from build123d import *

# Parameters (mm, degrees)
CROQUIS4_R                  = 2.5
SALIENTE_EXTRUIR1_DEPTH     = 4
CROQUIS5_R                  = 21
SALIENTE_EXTRUIR2_DEPTH     = 8.5
SALIENTE_EXTRUIR4_START     = -3
SALIENTE_EXTRUIR4_DEPTH     = 3
REDONDEO1_R                 = 10
SALIENTE_EXTRUIR5_OUTLINE_R = 2
SALIENTE_EXTRUIR5_DEPTH     = 15
CROQUIS9_R                  = 1.6
CORTAR_EXTRUIR1_DEPTH       = 70.417217007
CROQUIS11_W                 = 35
CROQUIS11_H                 = 53
SALIENTE_EXTRUIR7_DEPTH     = 7
CROQUIS12_W                 = 35
CROQUIS12_H                 = 7
SALIENTE_EXTRUIR8_DEPTH     = 28
CHAFL_N2_SIZE               = 7
CROQUIS13_R                 = 11.4
CORTAR_EXTRUIR2_DEPTH       = 2


# Read off the part's stored shape, not the designer's step: Saliente-Extruir5
with BuildPart() as part:
    # Croquis4 → Saliente-Extruir1 (new body)
    with BuildSketch(Plane.XY):
        with BuildLine():
            Line((-17.5, 27.5), (17.5, 27.5))
            ThreePointArc((17.5, 27.5), (24.571067812, 24.571067812), (27.5, 17.5))
            Line((27.5, 17.5), (27.5, -17.5))
            ThreePointArc((27.5, -17.5), (24.571067812, -24.571067812), (17.5, -27.5))
            Line((17.5, -27.5), (-17.5, -27.5))
            ThreePointArc((-17.5, -27.5), (-24.571067812, -24.571067812), (-27.5, -17.5))
            Line((-27.5, -17.5), (-27.5, 17.5))
            ThreePointArc((-27.5, 17.5), (-24.571067812, 24.571067812), (-17.5, 27.5))
        make_face()
        Circle(CROQUIS4_R, mode=Mode.SUBTRACT)
    extrude(amount=SALIENTE_EXTRUIR1_DEPTH)

    # Croquis5 → Saliente-Extruir2 (add)
    with BuildSketch(Plane.XY.offset(4)):
        with BuildLine():
            Line((-17.5, 27.5), (17.5, 27.5))
            ThreePointArc((17.5, 27.5), (24.571067812, 24.571067812), (27.5, 17.5))
            Line((27.5, 17.5), (27.5, -17.5))
            ThreePointArc((27.5, -17.5), (24.571067812, -24.571067812), (17.5, -27.5))
            Line((17.5, -27.5), (-17.5, -27.5))
            ThreePointArc((-17.5, -27.5), (-24.571067812, -24.571067812), (-27.5, -17.5))
            Line((-27.5, -17.5), (-27.5, 17.5))
            ThreePointArc((-27.5, 17.5), (-24.571067812, 24.571067812), (-17.5, 27.5))
        make_face()
        Circle(CROQUIS5_R, mode=Mode.SUBTRACT)
    extrude(amount=SALIENTE_EXTRUIR2_DEPTH)

    # Croquis6 → Saliente-Extruir4 (add)
    with BuildSketch(Plane.XY.offset(12.5).offset(SALIENTE_EXTRUIR4_START)):
        with BuildLine():
            Line((-25.720640569, -23.193950178), (-15, -57.5))
            Line((-15, -57.5), (15, -57.5))
            Line((15, -57.5), (25.720640569, -23.193950178))
            ThreePointArc((25.720640569, -23.193950178), (22.140069947, -26.358315353), (17.5, -27.5))
            Line((17.5, -27.5), (-17.5, -27.5))
            ThreePointArc((-17.5, -27.5), (-22.140069947, -26.358315353), (-25.720640569, -23.193950178))
        make_face()
    extrude(amount=SALIENTE_EXTRUIR4_DEPTH)

    # Redondeo1
    # the kernel refuses this fillet: 10 mm, written as the material it adds along each edge
    with BuildSketch(Plane(origin=(17.5, -17.5, 9.5), x_dir=(-0.31521717271258337, 0.949019564617656, 0), z_dir=(-0.949019564617656, -0.31521717271258337, 0))) as redondeo1_piece_1_section:
        with BuildLine():
            CenterArc((19.987492178, 10), REDONDEO1_R, 182.865983983, 87.134016017)
            Line((19.987492178, 0), (10, 0))
            Line((10, 0), (10, 9.5))
        make_face()
    redondeo1_piece_1 = revolve(axis=Axis((17.5, -17.5, 9.5), (0, 0, -1)), revolution_arc=198.373924806, mode=Mode.PRIVATE)
    redondeo1_piece_1 = split(redondeo1_piece_1, bisect_by=Plane(origin=(27.5, -26.624186886, 2.060383814), z_dir=(-1, 0, 0)), keep=Keep.TOP, mode=Mode.PRIVATE)
    redondeo1_piece_1 = redondeo1_piece_1 - Plane(origin=(0, 0, 2.060383814), x_dir=(1, 0, 0), z_dir=(0, 0, -1)) * Cylinder(21, 80, mode=Mode.PRIVATE)
    redondeo1_piece_1 = split(redondeo1_piece_1, bisect_by=Plane(origin=(24.437894836, -27.298736526, 2.060383814), z_dir=(-0.9544799780350299, 0.2982749931359464, 0)), keep=Keep.TOP, mode=Mode.PRIVATE)
    add(redondeo1_piece_1)
    with BuildSketch(Plane(origin=(-17.5, -17.5, 9.5), x_dir=(0, -1, 0), z_dir=(1, 0, 0))) as redondeo1_piece_2_section:
        with BuildLine():
            CenterArc((19.987492178, 10), REDONDEO1_R, 182.865983983, 87.134016017)
            Line((19.987492178, 0), (10, 0))
            Line((10, 0), (10, 9.5))
        make_face()
    redondeo1_piece_2 = revolve(axis=Axis((-17.5, -17.5, 9.5), (0, 0, -1)), revolution_arc=198.373924806, mode=Mode.PRIVATE)
    redondeo1_piece_2 = split(redondeo1_piece_2, bisect_by=Plane(origin=(-27.5, -26.624186886, 2.060383814), z_dir=(1, 0, 0)), keep=Keep.TOP, mode=Mode.PRIVATE)
    redondeo1_piece_2 = redondeo1_piece_2 - Plane(origin=(0, 0, 2.060383814), x_dir=(1, 0, 0), z_dir=(0, 0, -1)) * Cylinder(21, 80, mode=Mode.PRIVATE)
    redondeo1_piece_2 = split(redondeo1_piece_2, bisect_by=Plane(origin=(-24.437894836, -27.298736526, 2.060383814), z_dir=(0.9544799780350299, 0.29827499313594635, 0)), keep=Keep.TOP, mode=Mode.PRIVATE)
    add(redondeo1_piece_2)
    with BuildSketch(Plane(origin=(17.5, -27.5, 9.5), x_dir=(0, 0, -1), z_dir=(-1, 0, 0))) as redondeo1_piece_3:
        with BuildLine():
            CenterArc((10, 9.987492178), REDONDEO1_R, 180, 87.134016017)
            Line((0, 9.987492178), (0, 0))
            Line((0, 0), (9.5, 0))
        make_face()
    extrude(amount=35)

    # Saliente-Extruir5 outline → Saliente-Extruir5 (add)
    with BuildSketch(Plane.XY.offset(12.5)):
        with BuildLine():
            ThreePointArc((-27.5, -17.5), (-27.04479978, -20.482749931), (-25.720640569, -23.193950178))
            Line((-25.720640569, -23.193950178), (-15, -57.5))
            Line((-15, -57.5), (-12.5, -57.5))
            Line((-12.5, -57.5), (-12.5, -55.5))
            Line((-12.5, -55.5), (-15, -55.5))
            Line((-15, -55.5), (-15, -25))
            Line((-15, -25), (-11.560632513, -25))
            Line((-11.560632513, -25), (-11.560632513, -24.25))
            Line((-11.560632513, -24.25), (-22.25, -24.25))
            ThreePointArc((-22.25, -24.25), (-25.19427191, -20.722135955), (-26.25, -16.25))
            Line((-26.25, -16.25), (-26.25, 16.25))
            ThreePointArc((-26.25, 16.25), (-26.205571214, 17.191595354), (-26.072679638, 18.12482392))
            ThreePointArc((-26.072679638, 18.12482392), (-24.934779512, 19.680078923), (-23.010409798, 19.782235789))
            ThreePointArc((-23.010409798, 19.782235789), (-20.782444846, 20.273260806), (-20.464111601, 22.532375088))
            ThreePointArc((-20.464111601, 22.532375088), (-20.519074057, 24.539569231), (-19.008189542, 25.862096049))
            ThreePointArc((-19.008189542, 25.862096049), (-17.64266642, 26.152549179), (-16.25, 26.25))
            Line((-16.25, 26.25), (16.25, 26.25))
            ThreePointArc((16.25, 26.25), (17.64266642, 26.152549179), (19.008189542, 25.862096049))
            ThreePointArc((19.008189542, 25.862096049), (20.519074057, 24.539569231), (20.464111601, 22.532375088))
            ThreePointArc((20.464111601, 22.532375088), (20.782444846, 20.273260806), (23.010409798, 19.782235789))
            ThreePointArc((23.010409798, 19.782235789), (24.934779512, 19.680078923), (26.072679638, 18.12482392))
            ThreePointArc((26.072679638, 18.12482392), (26.205571214, 17.191595354), (26.25, 16.25))
            Line((26.25, 16.25), (26.25, -16.25))
            ThreePointArc((26.25, -16.25), (25.19427191, -20.722135955), (22.25, -24.25))
            Line((22.25, -24.25), (11.560632513, -24.25))
            Line((11.560632513, -24.25), (11.560632513, -25))
            Line((11.560632513, -25), (15, -25))
            Line((15, -25), (15, -55.5))
            Line((15, -55.5), (12.5, -55.5))
            Line((12.5, -55.5), (12.5, -57.5))
            Line((12.5, -57.5), (15, -57.5))
            Line((15, -57.5), (25.720640569, -23.193950178))
            ThreePointArc((25.720640569, -23.193950178), (27.04479978, -20.482749931), (27.5, -17.5))
            Line((27.5, -17.5), (27.5, 17.5))
            ThreePointArc((27.5, 17.5), (24.571067812, 24.571067812), (17.5, 27.5))
            Line((17.5, 27.5), (-17.5, 27.5))
            ThreePointArc((-17.5, 27.5), (-24.571067812, 24.571067812), (-27.5, 17.5))
            Line((-27.5, 17.5), (-27.5, -17.5))
        make_face()
        with Locations((-18, -36.75)):
            Circle(SALIENTE_EXTRUIR5_OUTLINE_R, mode=Mode.SUBTRACT)
        with Locations((18, -36.75)):
            Circle(SALIENTE_EXTRUIR5_OUTLINE_R, mode=Mode.SUBTRACT)
    extrude(amount=SALIENTE_EXTRUIR5_DEPTH)

    # Croquis9 → Cortar-Extruir1 (cut, through all)
    with BuildSketch(Plane.XY.offset(27.5)):
        with Locations((-22.25, 21.632040357)):
            Circle(CROQUIS9_R)
        with Locations((-18, -36.75)):
            Circle(CROQUIS9_R)
        with Locations((18, -36.75)):
            Circle(CROQUIS9_R)
        with Locations((22.25, 21.632040357)):
            Circle(CROQUIS9_R)
    extrude(amount=-CORTAR_EXTRUIR1_DEPTH, mode=Mode.SUBTRACT)

    # Croquis11 → Saliente-Extruir7 (add)
    with BuildSketch(Plane(origin=(0, 27.5, 0), x_dir=(1, 0, 0), z_dir=(0, 1, 0))):
        with Locations((0, -11.5)):
            Rectangle(CROQUIS11_W, CROQUIS11_H)
    extrude(amount=SALIENTE_EXTRUIR7_DEPTH)

    # Croquis12 → Saliente-Extruir8 (add)
    with BuildSketch(Plane.XZ.offset(-27.5)):
        with Locations((0, 41.5)):
            Rectangle(CROQUIS12_W, CROQUIS12_H)
        with Locations((0, -18.5)):
            Rectangle(CROQUIS12_W, CROQUIS12_H)
    extrude(amount=-SALIENTE_EXTRUIR8_DEPTH)

    # Chaflán2
    chafl_n2_edges = [part.edges().sort_by_distance(p)[0] for p in [
        (0, 27.5, 0),
    ]]
    chamfer(chafl_n2_edges, length=CHAFL_N2_SIZE)

    # Croquis13 → Cortar-Extruir2 (cut)
    with BuildSketch(Plane(origin=(0, 0, 0), x_dir=(-1, 0, 0), z_dir=(0, 0, -1))):
        Circle(CROQUIS13_R)
    extrude(amount=-CORTAR_EXTRUIR2_DEPTH, mode=Mode.SUBTRACT)


solid = part.part
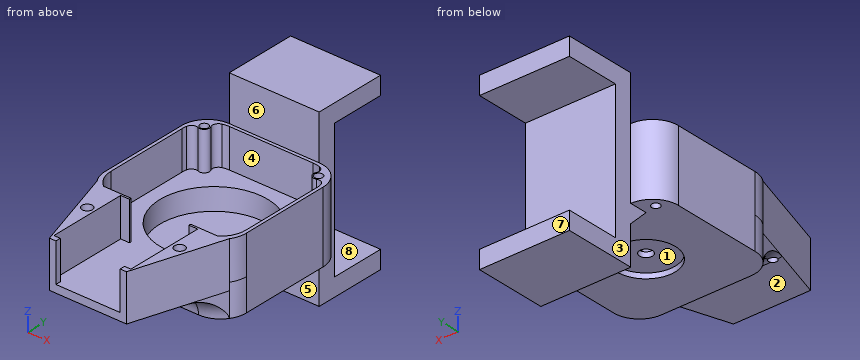
The listing builds one solid part. Answer for the finished solid, in the listing's coordinates (mm). Face numbers are marked on the shaded views. A direction names the side the tool comes from. Coordinates: 2 decimals unless noted, no trailing zeros. Write each loop counter-clockwise with the first axis right and the second up, starting at its lowest first coordinate (ties: lowest second). Pieces come first, ordered by that corner, then holes. Notation, with made-up numbers: M 21.25,31.5 L 29.25,31.5 A10 ccw 29.25,39.5 Z; hole C 23,-15 d2. An arc over 180 degrees is marked long. Put each result on its own line as item: value. Start each with the question number.
1. Which of the six approach directions +Z, -Z, +X, -X, +Y, -Y give full straight-line access (tool end or side, diameter ignored) to the marked faces 4, 5, 6, 7 and 8?
2. For a pull along X with two mould halves and no side action, classify the marked faces 1, 2 and 3 as pulls with the +X half, pulls with the -X half, needs draft (parallel to the pull), parting line crosses it, or undercut.
3. A cutting plane is placed at B-B on y = 0. Write down the section's boundary in (x, z), then the cut area to 3 significant figures.
4. Flat-ended cylindrical pins translate along their axes: P1, Ø12, axis at y = -44.5, z = 20, coming from the -X side; P2, Ø3, axis at x = -18, y = -36.75, coming from the -Z side; P3, Ø1.5, axis at x = -19, y = -41.5, coming from the -Z side; P4, Ø1, axis at y = -56.5, z = 23, coming from the +X side. Find the tip coordinate at first contact, or state that the pin passes through.
5. Consider line 1 (Z direction, x = -5.5, y = 49); line 2 (X direction, y = -36.75, z = 11.75); line 3 (Z direction, x = -18.5, y = -40.5). Determine where each line is inside the solid, lowest interval first. Write a range as from..to.
6. A cutting plane is placed at D-D on y = 14.5. Write down the section's boundary in (x, z).
7. A cutting plane is placed at C-C on z = 8. Write down the section's boundary in (x, y).
Resolved:
1. face 4: +Z
1. face 5: -Z, +X, -X, -Y
1. face 6: +Z, +X, -X, -Y
1. face 7: +Z, -Z, +X, -X, +Y
1. face 8: +X, -X, +Y
2. face 1: undercut
2. face 2: needs draft
2. face 3: pulls with the -X half
3. outline: M -27.5,0 L -11.4,0 L -11.4,2 L -2.5,2 L -2.5,4 L -21,4 L -21,12.5 L -26.25,12.5 L -26.25,27.5 L -27.5,27.5 Z; M 2.5,2 L 11.4,2 L 11.4,0 L 27.5,0 L 27.5,27.5 L 26.25,27.5 L 26.25,12.5 L 21,12.5 L 21,4 L 2.5,4 Z
3. area: 312 mm2
4. P1: stops at x = -20.94
4. P2: passes through
4. P3: stops at z = 9.5
4. P4: stops at x = 15.47
5. line 1: z = -22..-15, 38..45
5. line 2: x = -21.48..-19.6, -16.4..16.4, 19.6..21.48
5. line 3: z = 9.5..27.5
6. outline: M -27.5,0 L 27.5,0 L 27.5,27.5 L 26.25,27.5 L 26.25,12.5 L 15.19,12.5 L 15.19,4 L -15.19,4 L -15.19,12.5 L -26.25,12.5 L -26.25,27.5 L -27.5,27.5 Z
7. outline: M -27.5,-17.5 A10 ccw -25.72,-23.19 L -23.27,-31.04 A14.72 ccw -17.5,-32.22 L 17.5,-32.22 A14.72 ccw 23.27,-31.04 L 25.72,-23.19 A10 ccw 27.5,-17.5 L 27.5,17.5 A10 ccw 17.5,27.5 L 17.5,34.5 L -17.5,34.5 L -17.5,27.5 A10 ccw -27.5,17.5 Z; hole C -22.25,21.63 d3.2; hole C 0,0 d42; hole C 22.25,21.63 d3.2
